Input: part model. Units: mm. Frame: model coordinates. Face numbers are marked on the shaded views. A direction names the side the tool comes from. Coordinates: 2 decimals unless noted, no trailing zeros. Write each loop counter-clockwise with the first axis right and the second up, starting at its lowest first coordinate (ties: lowest second). Pieces come first, ordered by that corner, then holes. Notation, with made-up numbers: (50.25, -23) - (107.25, -23) arc R9 cw to (107.25, -8) - close; hole circle Ø4 at (-20.5, 24). An arc over 180 degrees is marked (long way). One line per question, with ' | ' between items. Start each with the question number.
1) Section query A-A on y = 33. Return loops of the section in (x, z).
2) First-contact query: P1, Ø10.5, axis at x = 68.5, y = 18.5, coming from the -Z side; P2, Ø5, axis at y = 30.5, z = -46.5, coming from the -X side; P3, Ø17.5, axis at y = 16, z = -54, coming from the +X side. Flat tips, straight axial feed; report the tip coordinate or a pass-through.
3) Section query B-B on x = 100. Return loops of the section in (y, z).
4) Section query C-C on z = -42. Return loops of the section in (x, y).
5) Reachability of the marked faces 1, 2, 3, 4 and 5 from +Z, -Z, +X, -X, +Y, -Y: full face, straight path, thin tool, end or side. Return the list, or none.
6) Line query: line 1 (X direction, y = 16, z = -42); line 2 (Z direction, x = 94.5, y = 16.5); line 3 (X direction, y = 20, z = -40). Output: solid intervals per line, ascending.
7) Draft query along X for the marked faces 6, 7 and 8. Return one class per face: released by +X, released by -X, zero draft, split by the parting line, or undercut.
8) Section query D-D on x = 31.6. Return loops of the section in (y, z), and give its area (3 significant figures).
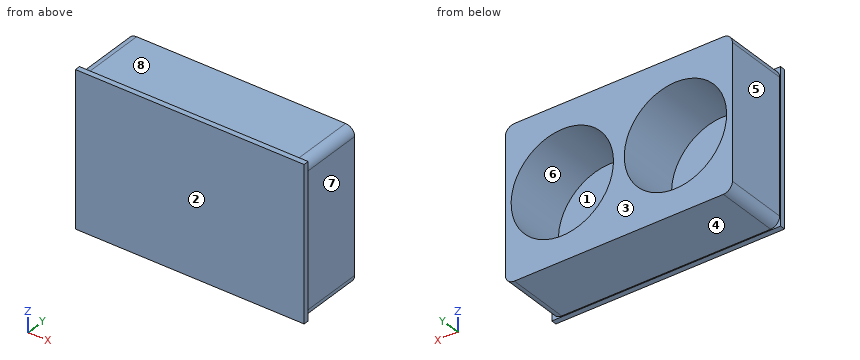
```python
from build123d import *

# Parameters (mm, degrees)
SKETCH2_W           = 126
SKETCH2_H           = 84
SKETCH2_R           = 28.4
BOSS_EXTRUDE1_DEPTH = 35
SKETCH3_W           = 127
SKETCH3_H           = 85
BOSS_EXTRUDE2_DEPTH = 3
FILLET1_R           = 5


with BuildPart() as part:
    # Sketch2 → Boss-Extrude1 (new body)
    with BuildSketch(Plane(origin=(0, 0, 0), x_dir=(1, 0, 0), z_dir=(0, 1, 0))):
        with Locations((63, 42)):
            Rectangle(SKETCH2_W, SKETCH2_H)
        with Locations(Location((31.6, 42, 0), (0, 0, 270))):
            Circle(SKETCH2_R, mode=Mode.SUBTRACT)
        with Locations(Location((94.4, 42, 0), (0, 0, 270))):
            Circle(SKETCH2_R, mode=Mode.SUBTRACT)
    extrude(amount=BOSS_EXTRUDE1_DEPTH)

    # Sketch3 → Boss-Extrude2 (add)
    with BuildSketch(Plane.XZ):
        with Locations((63, -42)):
            Rectangle(SKETCH3_W, SKETCH3_H)
    extrude(amount=BOSS_EXTRUDE2_DEPTH)

    # Fillet1
    fillet1_edges = [part.edges().sort_by_distance(p)[0] for p in [
        (0, 17.5, -84),
        (126, 17.5, -84),
        (126, 17.5, 0),
        (0, 17.5, 0),
    ]]
    fillet(fillet1_edges, radius=FILLET1_R)


solid = part.part
```
Answer key:
1) outline: (0, -79) arc R5 ccw to (5, -84) - (121, -84) arc R5 ccw to (126, -79) - (126, -5) arc R5 ccw to (121, 0) - (5, 0) arc R5 ccw to (0, -5) - close; hole circle Ø56.8 at (31.6, -42); hole circle Ø56.8 at (94.4, -42)
2) P1: z = -84 | P2: x = 0 | P3: x = 126
3) outline: (-3, -84.5) - (0, -84.5) - (0, -84) - (35, -84) - (35, -69.84) - (0, -69.84) - (0, -14.16) - (35, -14.16) - (35, 0) - (0, 0) - (0, 0.5) - (-3, 0.5) - close
4) outline: (-0.5, -3) - (126.5, -3) - (126.5, 0) - (126, 0) - (126, 35) - (122.8, 35) - (122.8, 0) - (66, 0) - (66, 35) - (60, 35) - (60, 0) - (3.2, 0) - (3.2, 35) - (0, 35) - (0, 0) - (-0.5, 0) - close
5) face 1: +Y | face 2: +Z, -Z, +X, -X, -Y | face 3: +Z, -Z, +X, -X, +Y | face 4: -Z, +X, -X, +Y | face 5: +Z, -Z, -X, +Y
6) line 1: 0 to 3.2, 60 to 66, 122.8 to 126 | line 2: -84 to -70.4, -13.6 to 0 | line 3: 0 to 3.27, 59.93 to 66.07, 122.73 to 126
7) face 6: undercut | face 7: released by +X | face 8: zero draft
8) outline: (-3, -84.5) - (0, -84.5) - (0, -84) - (35, -84) - (35, -70.4) - (0, -70.4) - (0, -13.6) - (35, -13.6) - (35, 0) - (0, 0) - (0, 0.5) - (-3, 0.5) - close | area: 1,210 mm²
